Geometry check sheet. Reference: the model listing, model coordinates, mm. A direction names the side the tool comes from. Give positions to 0.01 mm unless a question says otherwise; leave off trailing zeros. Order: outer loops, then holes, each group sorted by start corner. A loop starts at its lowest first (then second) coordinate and runs counter-clockwise, first axis right, second up. Notation, with made-up numbers: M -28.5,86.5 L 13.5,86.5 A27 ccw 13.5,104.5 Z; hole C 67.25,55 d2. An arc over 180 degrees is marked long. Answer as a JSON object with one key per item and string values. Group by question number.
from build123d import *

# Parameters (mm, degrees)
F0_W     = 40
F0_H     = 100
F1_DEPTH = 15
F3_DEPTH = 10
F4_W     = 100
F4_H     = 15
F5_DEPTH = 100


with BuildPart() as f1:
    # F0 (on Top) → F1 (new body)
    with BuildSketch(Plane.XY):
        Rectangle(F0_W, F0_H)
    extrude(amount=F1_DEPTH)

    # F2 (on face) → F3 (join)
    with BuildSketch(Plane(origin=(0, 0, 0), x_dir=(1, 0, 0), z_dir=(0, 0, -1))):
        Polygon((7.071068, 42.928932), (0, 50), (-7.071068, 42.928932), (-2.357023, 38.214887), (-4.714045, 35.857864), (-2.464045, 33.607864), (-4.714045, 31.357864), (-2.464045, 29.107864), (-4.714045, 26.857864), (-7.071068, 29.214887), (-11.785113, 24.500842), (-14.142136, 26.857864), (-18.856181, 22.143819), (-14.142136, 17.429774), (-11.785113, 19.786797), (-9.42809, 17.429774), (-7.071068, 19.786797), (-4.714045, 17.429774), (-7.071068, 15.072751), (-4.714045, 12.715729), (-6.964045, 10.465729), (-4.714045, 8.215729), (-6.964045, 5.965729), (-4.714045, 3.715729), (-6.964045, 1.465729), (-4.714045, -0.784271), (-6.964045, -3.034271), (-4.714045, -5.284271), (-6.964045, -7.534271), (-4.714045, -9.784271), (-6.964045, -12.034271), (-4.714045, -14.284271), (-6.964045, -16.534271), (-4.714045, -18.784271), (-6.964045, -21.034271), (-4.714045, -23.284271), (-7.071068, -25.641294), (0, -32.712362), (7.071068, -25.641294), (4.714045, -23.284271), (6.964045, -21.034271), (4.714045, -18.784271), (6.964045, -16.534271), (4.714045, -14.284271), (6.964045, -12.034271), (4.714045, -9.784271), (6.964045, -7.534271), (4.714045, -5.284271), (6.964045, -3.034271), (4.714045, -0.784271), (6.964045, 1.465729), (4.714045, 3.715729), (6.964045, 5.965729), (4.714045, 8.215729), (6.964045, 10.465729), (4.714045, 12.715729), (7.071068, 15.072751), (4.714045, 17.429774), (7.071068, 19.786797), (9.42809, 17.429774), (11.785113, 19.786797), (14.142136, 17.429774), (18.856181, 22.143819), (14.142136, 26.857864), (11.785113, 24.500842), (7.071068, 29.214887), (4.714045, 26.857864), (2.464045, 29.107864), (4.714045, 31.357864), (2.464045, 33.607864), (4.714045, 35.857864), (2.357023, 38.214887), align=None)
    extrude(amount=F3_DEPTH)

    # F4 (on face) → F5 (cut)
    with BuildSketch(Plane(origin=(-20, 0, 0), x_dir=(0, -1, 0), z_dir=(-1, 0, 0))):
        with Locations((0, 7.5)):
            Rectangle(F4_W, F4_H)
    extrude(amount=-F5_DEPTH, mode=Mode.SUBTRACT)


solid = f1.part
1. Access from +Z, -Z, +X, -X, +Y, -Y to the whole of each face (thin tool, end or side, straight path). Record for faces 4 (the flat face through (-5.9, -9.4, -4.9)), 5 (the flat face through (-12.98, -18.59, -4.93)), 6 (the flat face through (5.909, -28.053, -4.93)).
2. Cross-section at C-C (x = -15.5). Record the cut outline in (y, z), and give its area (3 significant figures).
3. Release check for a two-part mould opening along X. For faces 1 (the flat face through (-11, -19, -5)), 2 (the flat face through (5.855, -11.575, -4.93)), 3 (the flat face through (-3.605, -34.749, -4.93)) record: released by +X, released by -X, zero draft, split by the parting line, or undercut.
4. Cross-section at A-A (x = -6). State how many separate pieces and enclosed holes the cut face has, and give its area (3 significant figures).
5. Thickness scan on line 1 along Y through (x, z) = (-3, -1); line 2 along Y through (x, z) = (16.5, -3.25); line 3 along X through (y, z) = (-19, -7.75). Record the ranges inside material, lowest first. Write a range as [from, to].
6. Cross-section at B-B (y = 27). Record the cut outline in (x, z), and give its area (3 significant figures).
7. Depth check by flat-ended pin: pin 1 (6 mm diameter, centred on y = -12.5, z = -9, fed in from +X); pin 2 (1.5 mm diameter, centred on y = -25.5, z = -2.5, fed in from +X); pin 3 (1.5 mm diameter, centred on x = -1, z = -6, fed in from +Y). Enter the tip coordinate at first touch or a pass-through.
Report:
{
 "1": {"face 4": "+Z, -Z, -X", "face 5": "+Z, -Z, +Y", "face 6": "+Z, -Z"},
 "2": {"outline": "M -25.5,-10 L -18.79,-10 L -18.79,0 L -25.5,0 Z", "area": "67.1 mm2"},
 "3": {"face 1": "undercut", "face 2": "released by +X", "face 3": "released by -X"},
 "4": {"separate pieces": "12", "enclosed holes": "0", "area": "313 mm2"},
 "5": {"line 1": "y = [-47, -38.86], [-37.57, -34.14], [-33.07, -29.64], [-28.57, 29.71]", "line 2": "y = [-24.5, -19.79]", "line 3": "x = [-15.71, -12.57], [-11, -7.86], [-6.28, 6.28], [7.86, 11], [12.57, 15.71]"},
 "6": {"outline": "M -5.71,-10 L 5.71,-10 L 5.71,0 L -5.71,0 Z", "area": "114 mm2"},
 "7": {"pin 1": "stops at x = 7.07", "pin 2": "stops at x = 16.25", "pin 3": "stops at y = 32.46"}
}
